Verification items for the finished model (mm, model axes). A direction names the side the tool comes from. Give positions to 0.01 mm unless a question says otherwise; leave off trailing zeros. Order: outer loops, then holes, each group sorted by start corner. A loop starts at its lowest first (then second) coordinate and runs counter-clockwise, first axis right, second up. Notation, with made-up numbers: (44, 42.5) - (94, 42.5) arc R26 cw to (94, 58.5) - close; hole circle Ø2 at (52, 22). An arc over 180 degrees is marked (long way). Answer as a JSON object with one key per item and string values.
Autodesk Inventor part; units mm, degrees
ref_plane "Work Plane1" through (279.4, 0, 0) normal (1, 0, 0) x (0, 1, 0)
ref_plane "Work Plane2" through (-25.4, 0, 0) normal (1, 0, 0) x (0, 1, 0)
ref_plane "Work Plane3" through (127, 0, 0) normal (1, 0, 0) x (0, 1, 0)
sketch "Sketch1" plane through (0, 0, 0) normal (0, 0, 1) x (1, 0, 0)
  line L0 (0, 25.4) -> (254, 25.4)
  line L1 (254, 25.4) -> (254, -25.4)
  line L2 (254, -25.4) -> (0, -25.4)
  line L3 (0, -25.4) -> (0, 25.4)
  circle A0 centre (0, 0) radius 25.4
  circle A1 centre (254, 0) radius 25.4
  dimension "d0" = 254
  dimension "d1" = 50.8
extrude "Extrusion1" add sketch "Sketch1" along normal mid plane 50.8
sketch "Sketch2" plane through (0, 25.4, 25.4) normal (0, 1, 0) x (1, 0, 0)
  line L0 (-25.4, 50.8) -> (-25.4, 0)
  line L1 (-25.4, 50.8) -> (0, 50.8)
  line L2 (0, 0) -> (-25.4, 0)
  line L3 (0, 0) -> (254, 0)
  line L4 (254, 50.8) -> (0, 50.8)
  line L5 (-25.4, 12.7) -> (25.4, 12.7)
  line L6 (25.4, 12.7) -> (25.4, 38.1)
  line L7 (25.4, 38.1) -> (-25.4, 38.1)
  line L8 (-25.4, 38.1) -> (-25.4, 12.7)
  point P0 (-25.4, 25.4)
  point P1 (-25.4, 25.4)
  dimension "d4" = 25.4
  dimension "d10" = 50.8
extrude "Extrusion2" cut sketch "Sketch2" against normal through all
ref_plane "Work Plane1" through (279.4, 0, 0) normal (1, 0, 0) x (0, 1, 0)
ref_plane "Work Plane2" through (-25.4, 0, 0) normal (1, 0, 0) x (0, 1, 0)
ref_plane "Work Plane3" through (127, 0, 0) normal (1, 0, 0) x (0, 1, 0)
sketch "Sketch5" plane through (0, 0, 25.4) normal (0, 0, 1) x (1, 0, 0)
  arc A0 (254, -25.4) -> (254, 25.4) centre (254, 0) ccw
  line L0 (0, 25.4) -> (254, 25.4)
  arc A1 (0, 25.4) -> (0, -25.4) centre (0, 0) ccw
  line L1 (254, -25.4) -> (0, -25.4)
  circle A2 centre (0, 0) radius 25.4 construction
  circle A3 centre (254, 0) radius 25.4 construction
  line L2 (38.1, 25.4) -> (38.1, -25.4)
  line L3 (215.9, 25.4) -> (215.9, -25.4)
  dimension "d11" = 12.7
  dimension "d13" = 12.7
extrude "Extrusion4" cut sketch "Sketch5" against normal blind 3.175 contours L1 L2 L0 L3
pattern_circular "Circular Pattern1" count 4 over 360 about axis through (-10, 0, 0) along (1, 0, 0) of "Extrusion4"
mirror "Mirror1" about plane through (127, 0, 0) normal (1, 0, 0) of "Extrusion2"
sketch "Sketch3" plane through (0, 0, 25.4) normal (0, 0, 1) x (1, 0, 0)
  arc A0 (0, 25.4) -> (0, -25.4) centre (0, 0) ccw
  arc A1 (254, -25.4) -> (254, 25.4) centre (254, 0) ccw
  circle A2 centre (0, 0) radius 12.7
  circle A3 centre (254, 0) radius 12.7
  dimension "d7" = 25.4
extrude "Extrusion3" add sketch "Sketch3" along normal blind 3.175
mirror "Mirror2" about plane through (0, 0, 0) normal (0, 0, 1) of "Extrusion3"
equation "\"d13\" = d11"
(1) Section check D-D (x = 60.5). Record the cut outline in (y, z) (3 decimals), then the cut area to 3 significant figures.
Computed values:
{"outline": "(-22.225, -22.225) - (22.225, -22.225) - (22.225, 22.225) - (-22.225, 22.225) - close", "area": "1,980 mm²"}
(2) Section check A-A (x = 238). Record the cut outline in (y, z).
Computed values:
{"outline": "(-25.4, -25.4) - (25.4, -25.4) - (25.4, -12.7) - (-25.4, -12.7) - close; (-25.4, 12.7) - (25.4, 12.7) - (25.4, 25.4) - (-25.4, 25.4) - close"}
(3) Gauge pin test, flat ends, axial feed: pin 1 Ø1.5 at (x, z) = (124.5, -3.5) entering from +Y (3 decimals); pin 2 Ø4 at (x, y) = (232, -12) entering from +Z; pin 3 Ø2 at (y, z) = (14, -11.5) entering from -X. Record the tip position at first contact, or that the pin passes through.
Computed values:
{"pin 1": "stops at y = 22.225", "pin 2": "stops at z = 25.4", "pin 3": "stops at x = 25.4"}
(4) Section check B-B (z = 16). Record the cut outline in (x, y) (3 decimals).
Computed values:
{"outline": "(0, -25.4) - (38.1, -25.4) - (38.1, -22.225) - (215.9, -22.225) - (215.9, -25.4) - (254, -25.4) arc R25.4 ccw to (254, 25.4) - (215.9, 25.4) - (215.9, 22.225) - (38.1, 22.225) - (38.1, 25.4) - (0, 25.4) arc R25.4 ccw to start"}
(5) Section check C-C (y = -17). Record the cut outline in (x, z) (3 decimals).
Computed values:
{"outline": "(-18.872, -25.4) - (38.1, -25.4) - (38.1, -22.225) - (215.9, -22.225) - (215.9, -25.4) - (272.872, -25.4) - (272.872, -12.7) - (228.6, -12.7) - (228.6, 12.7) - (272.872, 12.7) - (272.872, 25.4) - (215.9, 25.4) - (215.9, 22.225) - (38.1, 22.225) - (38.1, 25.4) - (-18.872, 25.4) - (-18.872, 12.7) - (25.4, 12.7) - (25.4, -12.7) - (-18.872, -12.7) - close"}
(6) Release check for a two-part mould opening along X. For faces 1 (the flat face through (25.4, 0, 0)), 2 (the cylindrical face through (266.114, -3.815, 26.965)), 3 (the flat face through (227, -25.4, 0)) record: pulls with the +X half, pulls with the -X half, needs draft (parallel to the pull), parting line crosses it, or undercut.
Computed values:
{"face 1": "pulls with the -X half", "face 2": "undercut", "face 3": "needs draft"}
(7) Access from +Z, -Z, +X, -X, +Y, -Y to the whole of each face (thin tool, end or side, straight path). Record for faces 4 (the flat face through (240, 0, -25.4)), 5 (the cylindrical face through (-2.75, 12.4, 26.97)), 6 (the flat face through (126, 0, -22.225)).
Computed values:
{"face 4": "-Z", "face 5": "+Z", "face 6": "-Z, +Y, -Y"}
(8) Material ranges on line 1 along Z through (x, y) = (-7.5, 18.5); line 2 along Z through (x, y) = (39.5, -16.5) (3 decimals); line 3 along X through (y, z) = (21.5, 3), recorded low to high. Write a range as [from, to].
Computed values:
{"line 1": "z = [-25.4, -12.7], [12.7, 25.4]", "line 2": "z = [-22.225, 22.225]", "line 3": "x = [25.4, 228.6]"}
